from build123d import *

# Parameters (mm, degrees)
F1_DEPTH = 12.7
F3_DEPTH = 152.4
F5_W     = 317.5
F5_H     = 12.7
F6_DEPTH = 330.2
F8_W     = 317.5
F8_H     = 6.35
F9_DEPTH = 76.2


with BuildPart() as f1:
    # F0 (on Right) → F1 (new body)
    with BuildSketch(Plane.YZ):
        Polygon((0, 152.4), (0, 0), (304.8, 0), (360.269064, 152.4), align=None)
    extrude(amount=F1_DEPTH)

    # F2 (on face) → F3 (join)
    with BuildSketch(Plane.YZ.offset(12.7)):
        Polygon((429.142626, 360.194716), (353.511535, 152.4), (360.269064, 152.4), (435.109675, 358.022889), align=None)
        Polygon((353.511535, 152.4), (298.042471, 0), (304.8, 0), (360.269064, 152.4), align=None)
    extrude(amount=F3_DEPTH)

    # F4: F1 across face


with BuildPart() as f1_1:
    add(f1.part)
    add(f1.part.mirror(Plane(origin=(165.1, 366.770487, 179.554949), x_dir=(0, 1, 0), z_dir=(1, 0, 0))))

    # F5 (on Front) → F6 (join)
    with BuildSketch(Plane.XZ):
        with Locations((158.75, 82.55)):
            Rectangle(F5_W, F5_H)
    extrude(amount=-F6_DEPTH)

    # F8 (on face) → F9 (join)
    with BuildSketch(Plane(origin=(0, 0, 76.2), x_dir=(1, 0, 0), z_dir=(0, 0, -1))):
        with Locations((158.75, -3.175)):
            Rectangle(F8_W, F8_H)
    extrude(amount=F9_DEPTH)


solid = f1_1.part
Here's how the part is built. I have some questions about the finished solid (model axes, mm). A direction names the side the tool comes from. Coordinates: 2 decimals unless noted, no trailing zeros. Write each loop counter-clockwise with the first axis right and the second up, starting at its lowest first coordinate (ties: lowest second). Pieces come first, ordered by that corner, then holes.
1) Thinking about a two-plate mould opening in Z: for faces 1 (the face through (6, 183, 152.4)), 2 (the face through (167.234, 312.104, 38.633)), 3 (the face through (12.7, 174, 121)), which applies, +Z half, -Z half, draft (parallel to the pull), parting line (faces both ways), or undercut?
Filled in:
face 1: +Z half
face 2: undercut
face 3: draft
2) If we section it at C-C (z = 25): List the corners of the cut face in (x, y) for me.
Filled in:
outline: (0, 0) - (330.2, 0) - (330.2, 313.9) - (0, 313.9) - close; hole (12.7, 6.35) - (317.5, 6.35) - (317.5, 307.14) - (12.7, 307.14) - close
3) I'm going to push flat-ended pins straight in: pin 1 (8 mm diameter, centred on x = 227.5, z = 93, fed in from -Y); pin 2 (4 mm diameter, centred on x = 322, y = 213, fed in from +Z); pin 3 (5 mm diameter, centred on x = 37, z = 129.5, fed in from -Y); pin 4 (5 mm diameter, centred on y = 278, z = 45, fed in from -X). Where does each tip first touch, or does it pass through?
Filled in:
pin 1: stops at y = 330.44
pin 2: stops at z = 152.4
pin 3: stops at y = 344.27
pin 4: stops at x = 0
4) Which directions (+Z, -Z, +X, -X, +Y, -Y) give clear straight access to the entire face, cutting with the end or side of a thin tool? Please do faces 4 (the face through (163, 6.35, 39)), 5 (the face through (163, 163, 88.9)), 6 (the face through (0, 178, 75)).
Filled in:
face 4: -Z
face 5: +Z, -Y
face 6: +Z, -Z, -X, +Y, -Y
5) If I drill on line 1 (X direction, y = 58.5, z = 41.5); line 2 (Z direction, x = 297, y = 283); line 3 (Y direction, x = 101, z = 221), over which ranges is the centre line in solid material (lowest first)?
Filled in:
line 1: x = 0 to 12.7, 317.5 to 330.2
line 2: z = 76.2 to 88.9
line 3: y = 378.48 to 385.24
6) If we section it at B-B (x = 131): List the corners of the cut face in (y, z) for me.
Filled in:
outline: (0, 0) - (6.35, 0) - (6.35, 76.2) - (325.78, 76.2) - (298.04, 0) - (304.8, 0) - (435.11, 358.02) - (429.14, 360.19) - (330.2, 88.35) - (330.2, 88.9) - (0, 88.9) - close
7) If we section it at A-A (y = 172): List the corners of the cut face in (x, z) for me.
Filled in:
outline: (0, 0) - (12.7, 0) - (12.7, 76.2) - (317.5, 76.2) - (317.5, 0) - (330.2, 0) - (330.2, 152.4) - (317.5, 152.4) - (317.5, 88.9) - (12.7, 88.9) - (12.7, 152.4) - (0, 152.4) - close
8) If we section it at D-D (z = 129): List the corners of the cut face in (x, y) for me.
Filled in:
outline: (0, 0) - (12.7, 0) - (12.7, 344.99) - (317.5, 344.99) - (317.5, 0) - (330.2, 0) - (330.2, 351.75) - (0, 351.75) - close
